```python
from build123d import *

# Parameters (mm, degrees)
EXTRUDE_1_DEPTH     = 400
SKETCH_2_W          = 22
SKETCH_2_H          = 13
CUT_EXTRUDE_1_DEPTH = 401.562105047
SKETCH_3_R          = 3
CUT_EXTRUDE_2_DEPTH = 401.492197177


with BuildPart() as part:
    # Эскиз1 → Бобышка-Вытянуть1 (new body)
    with BuildSketch(Plane(origin=(0, 0, 0), x_dir=(0, 0, -1), z_dir=(1, 0, 0))):
        with BuildLine():
            Line((0, 0), (0, 15))
            Line((0, 15), (1, 15))
            ThreePointArc((1, 15), (1.707106781, 14.707106781), (2, 14))
            Line((2, 14), (2, 3))
            ThreePointArc((2, 3), (2.292893219, 2.292893219), (3, 2))
            Line((3, 2), (14, 2))
            ThreePointArc((14, 2), (14.707106781, 1.707106781), (15, 1))
            Line((15, 1), (15, 0))
            Line((15, 0), (0, 0))
        make_face()
    extrude(amount=EXTRUDE_1_DEPTH)

    # Эскиз2 → Вырез-Вытянуть1 (cut, through all)
    with BuildSketch(Plane.XY):
        with Locations((389, 8.5)):
            Rectangle(SKETCH_2_W, SKETCH_2_H)
        with Locations((11, 8.5)):
            Rectangle(SKETCH_2_W, SKETCH_2_H)
    extrude(amount=-CUT_EXTRUDE_1_DEPTH, mode=Mode.SUBTRACT)

    # Эскиз3 → Вырез-Вытянуть2 (cut, through all)
    with BuildSketch(Plane(origin=(0, 2, 0), x_dir=(1, 0, 0), z_dir=(0, 1, 0))):
        with Locations(Location((390, 7.5, 0), (0, 0, 270))):
            Circle(SKETCH_3_R)
        with Locations(Location((10, 7.5, 0), (0, 0, 270))):
            Circle(SKETCH_3_R)
    extrude(amount=-CUT_EXTRUDE_2_DEPTH, mode=Mode.SUBTRACT)


solid = part.part
```
Geometry: final body of the model. Coordinates: model frame, mm. A direction names the side the tool comes from. Round coordinates to 2 decimals unless told otherwise and drop trailing zeros. Order: outer loops, then holes, each group sorted by start corner. A loop starts at its lowest first (then second) coordinate and runs counter-clockwise, first axis right, second up. Notation, with made-up numbers: (29, 13) -> (63, 13) arc R14 ccw to (63, 32) -> close; hole circle Ø9 at (39, 89). An arc over 180 degrees is marked (long way). Write each question's results on one line, items separated by ' | '.
Q1. Section query A-A (z = -7.5). Output: boundary loops of the cut face in (x, y), and give its area (3 significant figures).
Response values:
outline: (0, 0) -> (7, 0) -> (7, 2) -> (0, 2) -> close; (13, 0) -> (387, 0) -> (387, 2) -> (13, 2) -> close; (393, 0) -> (400, 0) -> (400, 2) -> (393, 2) -> close | area: 776 mm²
Q2. Section query B-B (x = 297). Output: boundary loops of the cut face in (y, z).
Response values:
outline: (0, -15) -> (1, -15) arc R1 ccw to (2, -14) -> (2, -3) arc R1 cw to (3, -2) -> (14, -2) arc R1 ccw to (15, -1) -> (15, 0) -> (0, 0) -> close
Q3. Ray query, line 1 along X through (y, z) = (0.75, -7.5); line 2 along Z through (x, y) = (66.5, 4.5); line 3 along Y through (x, z) = (241, -4). Return the intervals inside material, ascending.
Response values:
line 1: 0 to 7, 13 to 387, 393 to 400 | line 2: -2 to 0 | line 3: 0 to 2
Q4. Access query for faces 1 (the face through (197, 0, -8)), 2 (the face through (198, 9, -2)). Directions: +Z, -Z, +X, -X, +Y, -Y. A direction counts if a zero-diameter tool reaches every point of the face in a straight line with its end or side. Return the directions, or none.
Response values:
face 1: +Z, -Z, +X, -X, -Y | face 2: -Z, +X, -X, +Y
Q5. Section query C-C (y = 7.5). Output: boundary loops of the cut face in (x, z), and give its area (3 significant figures).
Response values:
outline: (22, -2) -> (378, -2) -> (378, 0) -> (22, 0) -> close | area: 712 mm²
Q6. Pin query (flat end, axial travel): pin 1 Ø1 at (y, z) = (13.5, -2) entering from -X; pin 2 Ø1 at (x, y) = (231.5, 6) entering from -Z; pin 3 Ø4 at (x, y) = (74, 12) entering from +Z; pin 4 Ø1.5 at (y, z) = (11.5, -3) entering from +X. Return the tip coordinate at first contact, or that it passes through.
Response values:
pin 1: x = 22 | pin 2: z = -2 | pin 3: z = 0 | pin 4: through
